Input: part model. Units: mm. Frame: model coordinates. A direction names the side the tool comes from. Round coordinates to 2 decimals unless told otherwise and drop trailing zeros. Answer in a Markdown table with one row per item. Add a question column.
Q1. Section A-A, the plane x = 90.5. Give the number of separate pieces and of enclosed holes in the cut face, and give its area (3 significant figures).
Q2. Pin query (flat end, axial travel): pin 1 (4 mm diameter, centred on y = -2.5, z = 1.5, fed in from -X); pin 2 (6 mm diameter, centred on y = 2, z = 0.5, fed in from -X). Return the tip coordinate at first contact, or that it passes through.
Q3. Reachability of faces 1 (the face through (35.9, -2.2, -4.762)), 2 (the face through (31, -6.35, 3)) from +Z, -Z, +X, -X, +Y, -Y: full face, straight path, thin tool, end or side. Return the list, or none.
Q4. Mould query, pull axis Y, two halves, no side actions, for faces 3 (the face through (31.9, -2.2, 4.762)), 4 (the face through (31, 6.35, 3)), 5 (the face through (31.9, -4.762, 2.2)), 6 (the face through (254, 0, -6)). Classes: pulls with the +Y half, pulls with the -Y half, needs draft (parallel to the pull), parting line crosses it, or undercut.
Q5. Ray query, L1, parallel to Z at x = 116, y = 3; L2, parallel to Y at x = 227, z = -5.75 (3 decimals). Return the intervals inside material, ascending. Write a range as from..to.
```python
from build123d import *

# Parameters (mm, degrees)
BOSS_EXTRUDE1_DEPTH      = 254
BOSS_EXTRUDE1_DEPTH_BACK = 185.42
SKETCH1_W                = 12.7
SKETCH1_H                = 12.7
SKETCH1_W_2              = 9.525
SKETCH1_H_2              = 9.525
CUT_EXTRUDE1_DEPTH       = 255.158700422
CUT_EXTRUDE1_DEPTH_BACK  = 255.158700422
CUT_EXTRUDE2_DEPTH       = 255.396565425
CUT_EXTRUDE3_DEPTH       = 255.396565425


with BuildPart() as part:
    # Sketch1 → Boss-Extrude1 (new, two sides: drawn at the far end of the back side and taken through both)
    with BuildSketch(Plane(origin=(0, 0, 0), x_dir=(0, 0, -1), z_dir=(1, 0, 0)).offset(-BOSS_EXTRUDE1_DEPTH_BACK)):
        Rectangle(SKETCH1_W, SKETCH1_H)
        Rectangle(SKETCH1_W_2, SKETCH1_H_2, mode=Mode.SUBTRACT)
    extrude(amount=BOSS_EXTRUDE1_DEPTH + BOSS_EXTRUDE1_DEPTH_BACK)

    # Sketch2 → Cut-Extrude1 (cut, two sides: drawn at the far end of the back side and taken through both)
    with BuildSketch(Plane(origin=(0, 0, 0), x_dir=(1, 0, 0), z_dir=(0, 1, 0)).offset(-CUT_EXTRUDE1_DEPTH_BACK)):
        Polygon((-185.42, -6.35), (-174.250456919, 6.961343094), (-183.078216502, 14.368712905), (-194.247759583, 1.057369811), align=None)
    extrude(amount=CUT_EXTRUDE1_DEPTH + CUT_EXTRUDE1_DEPTH_BACK, mode=Mode.SUBTRACT)

    # Sketch3 → Cut-Extrude2 (cut, through all)
    with BuildSketch(Plane(origin=(0, 6.35, 0), x_dir=(1, 0, 0), z_dir=(0, 1, 0))):
        with BuildLine():
            Line((-114.3, 1.905), (-76.2, 1.905))
            ThreePointArc((-76.2, 1.905), (-74.295, 0), (-76.2, -1.905))
            Line((-76.2, -1.905), (-114.3, -1.905))
            ThreePointArc((-114.3, -1.905), (-116.205, 0), (-114.3, 1.905))
        make_face()
        with BuildLine():
            Line((-50.8, 1.905), (-12.7, 1.905))
            ThreePointArc((-12.7, 1.905), (-10.795, 0), (-12.7, -1.905))
            Line((-12.7, -1.905), (-50.8, -1.905))
            ThreePointArc((-50.8, -1.905), (-52.705, 0), (-50.8, 1.905))
        make_face()
        with BuildLine():
            Line((12.7, 1.905), (50.8, 1.905))
            ThreePointArc((50.8, 1.905), (52.705, 0), (50.8, -1.905))
            Line((50.8, -1.905), (12.7, -1.905))
            ThreePointArc((12.7, -1.905), (10.795, 0), (12.7, 1.905))
        make_face()
        with BuildLine():
            Line((76.2, 1.905), (114.3, 1.905))
            ThreePointArc((114.3, 1.905), (116.205, 0), (114.3, -1.905))
            Line((114.3, -1.905), (76.2, -1.905))
            ThreePointArc((76.2, -1.905), (74.295, 0), (76.2, 1.905))
        make_face()
        with BuildLine():
            Line((139.7, 1.905), (177.8, 1.905))
            ThreePointArc((177.8, 1.905), (179.705, 0), (177.8, -1.905))
            Line((177.8, -1.905), (139.7, -1.905))
            ThreePointArc((139.7, -1.905), (137.795, 0), (139.7, 1.905))
        make_face()
        with BuildLine():
            Line((203.2, 1.905), (241.3, 1.905))
            ThreePointArc((241.3, 1.905), (243.205, 0), (241.3, -1.905))
            Line((241.3, -1.905), (203.2, -1.905))
            ThreePointArc((203.2, -1.905), (201.295, 0), (203.2, 1.905))
        make_face()
    extrude(amount=-CUT_EXTRUDE2_DEPTH, mode=Mode.SUBTRACT)

    # Sketch4 → Cut-Extrude3 (cut, through all)
    with BuildSketch(Plane.XY.offset(6.35)):
        with BuildLine():
            Line((-114.3, 1.905), (-76.2, 1.905))
            ThreePointArc((-76.2, 1.905), (-74.295, 0), (-76.2, -1.905))
            Line((-76.2, -1.905), (-114.3, -1.905))
            ThreePointArc((-114.3, -1.905), (-116.205, 0), (-114.3, 1.905))
        make_face()
        with BuildLine():
            Line((-50.8, 1.905), (-12.7, 1.905))
            ThreePointArc((-12.7, 1.905), (-10.795, 0), (-12.7, -1.905))
            Line((-12.7, -1.905), (-50.8, -1.905))
            ThreePointArc((-50.8, -1.905), (-52.705, 0), (-50.8, 1.905))
        make_face()
        with BuildLine():
            Line((12.7, 1.905), (50.8, 1.905))
            ThreePointArc((50.8, 1.905), (52.705, 0), (50.8, -1.905))
            Line((50.8, -1.905), (12.7, -1.905))
            ThreePointArc((12.7, -1.905), (10.795, 0), (12.7, 1.905))
        make_face()
        with BuildLine():
            Line((76.2, 1.905), (114.3, 1.905))
            ThreePointArc((114.3, 1.905), (116.205, 0), (114.3, -1.905))
            Line((114.3, -1.905), (76.2, -1.905))
            ThreePointArc((76.2, -1.905), (74.295, 0), (76.2, 1.905))
        make_face()
        with BuildLine():
            Line((139.7, 1.905), (177.8, 1.905))
            ThreePointArc((177.8, 1.905), (179.705, 0), (177.8, -1.905))
            Line((177.8, -1.905), (139.7, -1.905))
            ThreePointArc((139.7, -1.905), (137.795, 0), (139.7, 1.905))
        make_face()
        with BuildLine():
            Line((203.2, 1.905), (241.3, 1.905))
            ThreePointArc((241.3, 1.905), (243.205, 0), (241.3, -1.905))
            Line((241.3, -1.905), (203.2, -1.905))
            ThreePointArc((203.2, -1.905), (201.295, 0), (203.2, 1.905))
        make_face()
    extrude(amount=-CUT_EXTRUDE3_DEPTH, mode=Mode.SUBTRACT)


solid = part.part
```
Answer block:
| question | item | result |
|---|---|---|
| 1 | separate pieces | 4 |
| 1 | enclosed holes | 0 |
| 1 | area | 46.4 mm^2 |
| 2 | pin 1 | through |
| 2 | pin 2 | x = -181.49 |
| 3 | face 1 | +X, -X |
| 3 | face 2 | +Z, -Z, +X, -X, -Y |
| 4 | face 3 | undercut |
| 4 | face 4 | pulls with the +Y half |
| 4 | face 5 | undercut |
| 4 | face 6 | needs draft |
| 5 | L1 | -6.35..-4.76, 4.76..6.35 |
| 5 | L2 | -6.35..-1.905, 1.905..6.35 |
